Check sheet for the modelled part. Datum: model origin and axes. Units: mm. Coordinates: 2 decimals unless noted, no trailing zeros. Write each loop counter-clockwise with the first axis right and the second up, starting at its lowest first coordinate (ties: lowest second). Pieces come first, ordered by that corner, then holes. Notation, with made-up numbers: (-30.5, -33.5) - (-10.5, -33.5) arc R10 cw to (-10.5, -17.5) - close; hole circle Ø6 at (70.5, 7.5). An arc over 180 degrees is marked (long way). Use one line per item in the form item = value. Start each with the question number.
1. Cross-section at B-B on y = 3.95. Record the boundary of the cut face in (x, z) (3 decimals), then the cut area to 3 significant figures.
2. Scan lines: line 1 along Y through (x, z) = (4, -0.05); line 2 along Y through (x, z) = (4.5, 0); line 3 along X through (y, z) = (2.75, 0.05). Record each from-to range of solid material in increasing order.
3. Cross-section at A-A on z = 0. Record the boundary of the cut face in (x, y).
4. Cross-section at C-C on x = 3.75. Record the boundary of the cut face in (y, z) (3 decimals), then the cut area to 3 significant figures.
5. Go/stop test with a flat-tipped pin: pin 1 Ø3 at (x, y) = (4.5, 2) entering from +Z (3 decimals). Record where the tip stops, or that it passes through.
```python
from build123d import *

# Parameters (mm, degrees)
BOSS_EXTRUDE1_DEPTH = 0.125
FILLET1_R           = 0.3


with BuildPart() as part:
    # frame_outline → Boss-Extrude1 (new, symmetric)
    with BuildSketch(Plane.XY):
        Polygon((0, 0), (0, 1.1), (0.5, 1.1), (0.5, 0.6), (0.75, 0.6), (0.75, 1.1), (1.294312935, 1.1), (6.832215904, 5.513992793), (6.832215904, 3.691761529), (1.294312935, 0), align=None)
    extrude(amount=BOSS_EXTRUDE1_DEPTH, both=True)

    # Fillet1
    fillet1_edges = [part.edges().sort_by_distance(p)[0] for p in [
        (0, 0, 0),
        (0, 1.1, 0),
    ]]
    fillet(fillet1_edges, radius=FILLET1_R)


solid = part.part
```
Final values:
q1.outline = (4.87, -0.125) - (6.832, -0.125) - (6.832, 0.125) - (4.87, 0.125) - close
q1.area = 0.491 mm²
q2.line_1 = 1.8 to 3.26
q2.line_2 = 2.14 to 3.66
q2.line_3 = 3.36 to 5.42
q3.outline = (0, 0.3) arc R0.3 ccw to (0.3, 0) - (1.29, 0) - (6.83, 3.69) - (6.83, 5.51) - (1.29, 1.1) - (0.75, 1.1) - (0.75, 0.6) - (0.5, 0.6) - (0.5, 1.1) - (0.3, 1.1) arc R0.3 ccw to (0, 0.8) - close
q4.outline = (1.637, -0.125) - (3.057, -0.125) - (3.057, 0.125) - (1.637, 0.125) - close
q4.area = 0.355 mm²
q5.pin_1 = 0.125
